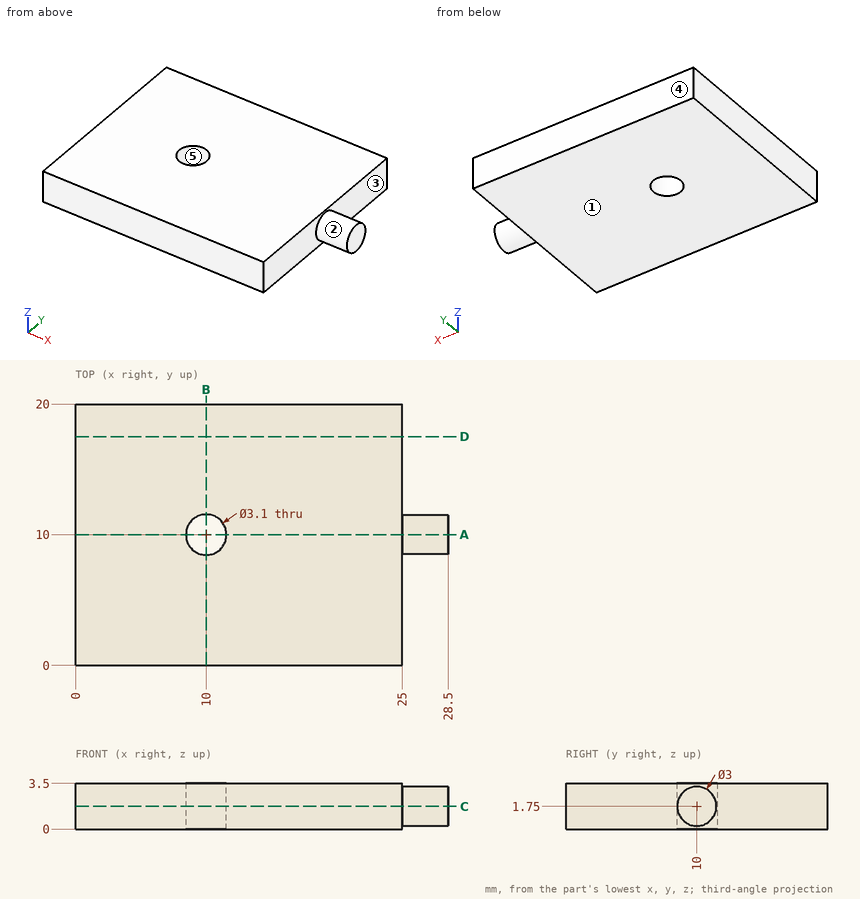
Check sheet for the drawn part. Datum: minimum x, y, z corner. Units: mm. A direction names the side the tool comes from. Round coordinates to 2 decimals unless told otherwise and drop trailing zeros. Loops run counter-clockwise (first coordinate to the right, second up) from the corner with the lowest first, then second, coordinate; pieces in that order, holes last. Notation, with made-up numbers: (46, -40) - (61, -40) arc R35 cw to (61, -2) - close; hole circle Ø5 at (-2, 5). An arc over 180 degrees is marked (long way). Write item = value, one per line. Start each with the question number.
1. Section check B-B on x = 10. Enter the section's corners in (y, z).
2. Thickness scan on line 1 (Y direction, x = 10, z = 0.8); line 2 (X direction, y = 14.5, z = 0.5). Record the ranges inside material, lowest first.
3. Section check C-C on z = 1.75. Enter the section's corners in (x, y), then the cut area to 3 significant figures.
4. Mould release check, pull along Y, two halves, no side actions. Record for the marked faces 3, 4 and 5: released by +Y, released by -Y, zero draft, split by the parting line, or undercut.
5. Section check D-D on y = 17.5. Enter the section's corners in (x, z).
6. Set-up check for the marked faces 1 and 2: record each of +Z, -Z, +X, -X, +Y, -Y from which the full face is reachable in a straight line by a thin tool's end or side.
7. Section check A-A on y = 10. Enter the section's corners in (x, z).
Working result:
q1.outline = (0, 0) - (8.45, 0) - (8.45, 3.5) - (0, 3.5) - close; (11.55, 0) - (20, 0) - (20, 3.5) - (11.55, 3.5) - close
q2.line_1 = 0 to 8.45, 11.55 to 20
q2.line_2 = 0 to 25
q3.outline = (0, 0) - (25, 0) - (25, 8.5) - (28.5, 8.5) - (28.5, 11.5) - (25, 11.5) - (25, 20) - (0, 20) - close; hole circle Ø3.1 at (10, 10)
q3.area = 503 mm^2
q4.face_3 = zero draft
q4.face_4 = released by +Y
q4.face_5 = undercut
q5.outline = (0, 0) - (25, 0) - (25, 3.5) - (0, 3.5) - close
q6.face_1 = -Z, +X, -X, +Y, -Y
q6.face_2 = +X
q7.outline = (0, 0) - (8.45, 0) - (8.45, 3.5) - (0, 3.5) - close; (11.55, 0) - (25, 0) - (25, 0.25) - (28.5, 0.25) - (28.5, 3.25) - (25, 3.25) - (25, 3.5) - (11.55, 3.5) - close
